```python
from build123d import *

# Parameters (mm, degrees)
SKETCH_1_W          = 62.2
SKETCH_1_H          = 78.2
SKETCH_1_W_2        = 59
SKETCH_1_H_2        = 75
EXTRUDE_1_DEPTH     = 30
SKETCH_2_W          = 62.2
SKETCH_2_H          = 78.2
EXTRUDE_1_2_DEPTH   = 1.6
SKETCH_3_W          = 5
SKETCH_3_H          = 5
EXTRUDE_2_DEPTH     = 3
SKETCH_4_W          = 1.5
SKETCH_4_H          = 5
EXTRUDE_3_DEPTH     = 1
SKETCH_5_W          = 1.5
SKETCH_5_H          = 5
SKETCH_5_H_2        = 4.722364884
EXTRUDE_4_DEPTH     = 1
FILLET_1_R          = 1
FILLET_2_R          = 1.8
SKETCH_6_R          = 2.2
CUT_EXTRUDE_1_DEPTH = 58.468078096
EXTRUDE_START       = 2
SKETCH_7_R          = 4
SKETCH_7_R_2        = 2.2
EXTRUDE_5_DEPTH     = 2
CHAMFER_1_SIZE      = 1.5
FILLET_3_R          = 1
CUT_EXTRUDE_2_REACH = 91.345


with BuildPart() as part:
    # Эскиз1 → Extrude 1 (new body)
    with BuildSketch(Plane.XY):
        Rectangle(SKETCH_1_W, SKETCH_1_H)
        Rectangle(SKETCH_1_W_2, SKETCH_1_H_2, mode=Mode.SUBTRACT)
    extrude(amount=EXTRUDE_1_DEPTH)

    # Эскиз2 → Extrude 1 2 (add)
    with BuildSketch(Plane.XY.offset(30)):
        Rectangle(SKETCH_2_W, SKETCH_2_H)
    extrude(amount=-EXTRUDE_1_2_DEPTH)

    # Эскиз3 → Бобышка-Вытянуть2 (add)
    with BuildSketch(Plane(origin=(0, 0, 28.4), x_dir=(-1, 0, 0), z_dir=(0, 0, -1))):
        with Locations((-27, 35)):
            Rectangle(SKETCH_3_W, SKETCH_3_H)
        with Locations((27, 35)):
            Rectangle(SKETCH_3_W, SKETCH_3_H)
        with Locations((-27, -35)):
            Rectangle(SKETCH_3_W, SKETCH_3_H)
        with Locations((27, -35)):
            Rectangle(SKETCH_3_W, SKETCH_3_H)
    extrude(amount=EXTRUDE_2_DEPTH)

    # Эскиз4 → Бобышка-Вытянуть3 (add)
    with BuildSketch(Plane.ZY.offset(-29.5)):
        with Locations((23.15, 35)):
            Rectangle(SKETCH_4_W, SKETCH_4_H)
        with Locations((23.15, -35)):
            Rectangle(SKETCH_4_W, SKETCH_4_H)
    extrude(amount=EXTRUDE_3_DEPTH)

    # Эскиз5 → Бобышка-Вытянуть4 (add)
    with BuildSketch(Plane(origin=(-29.5, 0, 0), x_dir=(0, 0, -1), z_dir=(1, 0, 0))):
        with Locations((-23.15, 35)):
            Rectangle(SKETCH_5_W, SKETCH_5_H)
        with Locations((-23.15, -35.138817558)):
            Rectangle(SKETCH_5_W, SKETCH_5_H_2)
    extrude(amount=EXTRUDE_4_DEPTH)

    # Скругление1
    fillet_1_edges = [part.edges().sort_by_distance(p)[0] for p in [
        (27, 32.5, 28.4),
        (24.5, 35, 28.4),
        (27, 32.5, 25.4),
        (24.5, 35, 25.4),
        (-24.5, 35, 28.4),
        (-27, 32.5, 28.4),
        (-24.5, 35, 25.4),
        (-27, 32.5, 25.4),
        (24.5, -35, 28.4),
        (27, -32.5, 28.4),
        (24.5, -35, 25.4),
        (27, -32.5, 25.4),
        (-27, -32.5, 28.4),
        (-24.5, -35, 28.4),
        (-27, -32.5, 25.4),
        (-24.5, -35, 25.4),
    ]]
    fillet(fillet_1_edges, radius=FILLET_1_R)

    # Скругление2
    # the kernel refuses this fillet: 1.8 mm, written as the material it adds along each edge
    with BuildSketch(Plane(origin=(29.5, -41.531128874, 23.9), x_dir=(0, 0, 1), z_dir=(0, 1, 0))) as fillet_2_piece_1_section:
        with BuildLine():
            CenterArc((1.61245155, -1.8), FILLET_2_R, 90, 63.612200039)
            Line((0, -1), (0, 0))
            Line((0, 0), (1.61245155, 0))
        make_face()
    fillet_2_piece_1 = extrude(amount=9.031128874, mode=Mode.PRIVATE)
    fillet_2_piece_1 = split(fillet_2_piece_1, bisect_by=Plane(origin=(29.5, -39.1, 23.9), z_dir=(0, 1, 0)), keep=Keep.TOP, mode=Mode.PRIVATE)
    add(fillet_2_piece_1)
    with BuildSketch(Plane(origin=(-29.5, -32.777635116, 23.9), x_dir=(0, 0, 1), z_dir=(0, -1, 0))) as fillet_2_piece_2_section:
        with BuildLine():
            CenterArc((1.61245155, -1.8), FILLET_2_R, 90, 63.612200039)
            Line((0, -1), (0, 0))
            Line((0, 0), (1.61245155, 0))
        make_face()
    fillet_2_piece_2 = extrude(amount=8.753493758, mode=Mode.PRIVATE)
    fillet_2_piece_2 = split(fillet_2_piece_2, bisect_by=Plane(origin=(-29.5, -39.1, 23.9), z_dir=(0, 1, 0)), keep=Keep.TOP, mode=Mode.PRIVATE)
    add(fillet_2_piece_2)
    with BuildSketch(Plane(origin=(-29.5, 41.531128874, 23.9), x_dir=(0, 0, 1), z_dir=(0, -1, 0))) as fillet_2_piece_3_section:
        with BuildLine():
            CenterArc((1.61245155, -1.8), FILLET_2_R, 90, 63.612200039)
            Line((0, -1), (0, 0))
            Line((0, 0), (1.61245155, 0))
        make_face()
    fillet_2_piece_3 = extrude(amount=9.031128874, mode=Mode.PRIVATE)
    fillet_2_piece_3 = split(fillet_2_piece_3, bisect_by=Plane(origin=(-29.5, 39.1, 23.9), z_dir=(0, -1, 0)), keep=Keep.TOP, mode=Mode.PRIVATE)
    add(fillet_2_piece_3)
    with BuildSketch(Plane(origin=(29.5, 41.531128874, 23.9), x_dir=(0, 0, 1), z_dir=(0, -1, 0))) as fillet_2_piece_4_section:
        with BuildLine():
            CenterArc((1.61245155, 1.8), FILLET_2_R, 206.387799961, 63.612200039)
            Line((0, 1), (0, 0))
            Line((0, 0), (1.61245155, 0))
        make_face()
    fillet_2_piece_4 = extrude(amount=9.031128874, mode=Mode.PRIVATE)
    fillet_2_piece_4 = split(fillet_2_piece_4, bisect_by=Plane(origin=(29.5, 39.1, 23.9), z_dir=(0, -1, 0)), keep=Keep.TOP, mode=Mode.PRIVATE)
    add(fillet_2_piece_4)

    # Эскиз6 → Вырез-Вытянуть1 (cut, through all)
    with BuildSketch(Plane(origin=(0, 0, 28.4), x_dir=(-1, 0, 0), z_dir=(0, 0, -1))):
        with Locations((-19.5, 25)):
            Circle(SKETCH_6_R)
        with Locations((0.5, 25)):
            Circle(SKETCH_6_R)
        with Locations((0.5, -25)):
            Circle(SKETCH_6_R)
        with Locations((-19.5, -25)):
            Circle(SKETCH_6_R)
    extrude(amount=-CUT_EXTRUDE_1_DEPTH, mode=Mode.SUBTRACT)

    # Эскиз7 → Бобышка-Вытянуть5 (add)
    # profile 1 of 4: a face of its own
    with BuildSketch(Plane(origin=(0, 0, 28.4), x_dir=(-1, 0, 0), z_dir=(0, 0, -1)).offset(EXTRUDE_START)):
        with Locations(Location((-19.5, 25, 0), (0, 0, 180))):
            Circle(SKETCH_7_R)
        with Locations((-19.5, 25)):
            Circle(SKETCH_7_R_2, mode=Mode.SUBTRACT)
    # profile 2 of 4: a face of its own
    with BuildSketch(Plane(origin=(0, 0, 28.4), x_dir=(-1, 0, 0), z_dir=(0, 0, -1)).offset(EXTRUDE_START)):
        with Locations(Location((0.5, 25, 0), (0, 0, 180))):
            Circle(SKETCH_7_R)
        with Locations((0.5, 25)):
            Circle(SKETCH_7_R_2, mode=Mode.SUBTRACT)
    # profile 3 of 4: a face of its own
    with BuildSketch(Plane(origin=(0, 0, 28.4), x_dir=(-1, 0, 0), z_dir=(0, 0, -1)).offset(EXTRUDE_START)):
        with Locations(Location((-19.5, -25, 0), (0, 0, 180))):
            Circle(SKETCH_7_R)
        with Locations((-19.5, -25)):
            Circle(SKETCH_7_R_2, mode=Mode.SUBTRACT)
    # profile 4 of 4: a face of its own
    with BuildSketch(Plane(origin=(0, 0, 28.4), x_dir=(-1, 0, 0), z_dir=(0, 0, -1)).offset(EXTRUDE_START)):
        with Locations(Location((0.5, -25, 0), (0, 0, 180))):
            Circle(SKETCH_7_R)
        with Locations((0.5, -25)):
            Circle(SKETCH_7_R_2, mode=Mode.SUBTRACT)
    extrude(amount=-EXTRUDE_5_DEPTH)

    # Фаска1
    chamfer_1_edges = [part.edges().sort_by_distance(p)[0] for p in [
        (21.7, 25, 26.4),
        (1.7, 25, 26.4),
        (21.7, -25, 26.4),
        (1.7, -25, 26.4),
    ]]
    chamfer(chamfer_1_edges, length=CHAMFER_1_SIZE)

    # Скругление3
    fillet_3_edges = [part.edges().sort_by_distance(p)[0] for p in [
        (31.1, -39.1, 15),
        (-31.1, -39.1, 15),
        (-31.1, 39.1, 15),
        (31.1, 39.1, 15),
    ]]
    fillet(fillet_3_edges, radius=FILLET_3_R)

    # Эскиз8 → Вырез-Вытянуть2 (cut, up to next)
    with BuildSketch(Plane(origin=(0, 39.1, 0), x_dir=(1, 0, 0), z_dir=(0, 1, 0)), mode=Mode.PRIVATE) as cut_extrude_2_sk1:
        with BuildLine():
            Line((18.995015929, -25.968474999), (14.239793371, -25.968474999))
            ThreePointArc((14.239793371, -25.968474999), (12.517359829, -24.246041457), (14.239793371, -22.523607914))
            Line((14.239793371, -22.523607914), (18.995015929, -22.523607914))
            ThreePointArc((18.995015929, -22.523607914), (20.717449472, -24.246041457), (18.995015929, -25.968474999))
        make_face()
    cut_extrude_2_tool1 = extrude(cut_extrude_2_sk1.sketch, amount=-CUT_EXTRUDE_2_REACH, mode=Mode.PRIVATE) & part.part
    add(cut_extrude_2_tool1.solids().sort_by_distance((16.617405, 39.1, 24.246041))[0], mode=Mode.SUBTRACT)


solid = part.part
```
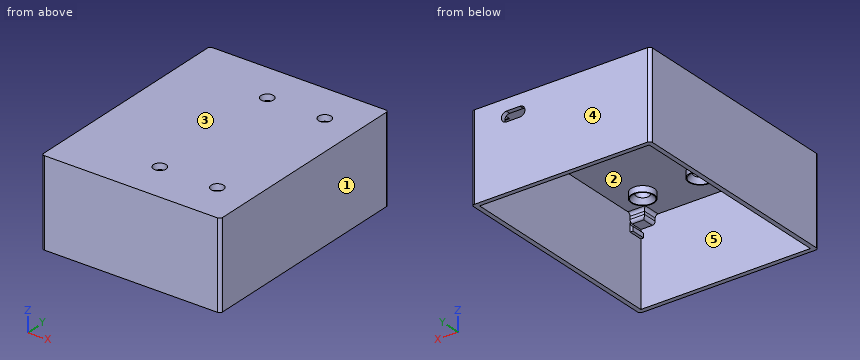
Verification items for the finished model (mm, model axes). Face numbers are marked on the shaded views. A direction names the side the tool comes from. Round coordinates to 2 decimals unless told otherwise and drop trailing zeros. Write each loop counter-clockwise with the first axis right and the second up, starting at its lowest first coordinate (ties: lowest second). Pieces come first, ordered by that corner, then holes.
1. Draft check along Y on the marked faces 3, 4 and 5. Enter one of: +Y half, -Y half, draft (parallel to the pull), parting line (faces both ways), or undercut.
2. Gauge pin test, flat ends, axial feed: P1, Ø2.5, axis at x = 19.5, y = -25, coming from the -Z side; P2, Ø0.5, axis at x = 29, y = 34, coming from the -Z side; P3, Ø4, axis at x = -0.5, y = -25.5, coming from the -Z side. Record the tip position at first contact, or that the pin passes through.
3. Section check B-B on x = -0.5. Enter the section's corners in (y, z), plus the area to 3 significant figures.
4. Scan lines: L1, parallel to Y at x = 19.5, z = 29.5; L2, parallel to X at y = -25.5, z = 12.25; L3, parallel to Y at x = -16, z = 10.25. Record each from-to range of solid material in increasing order.
5. Section check D-D on x = -13. Enter the section's corners in (y, z), plus the area to 3 significant figures.
6. Section check C-C on z = 20. Enter the section's corners in (x, y), plus the area to 3 significant figures.
7. Section check A-A on y = -25. Enter the section's corners in (x, z), plus the area to 3 significant figures.
8. Access from +Z, -Z, +X, -X, +Y, -Y to the whole of each face (thin tool, end or side, straight path). Record for the marked faces 1 and 2.
Answer:
1. face 3: draft
1. face 4: +Y half
1. face 5: undercut
2. P1: passes through
2. P2: stops at z = 22.4
2. P3: stops at z = 27.6
3. outline: (-39.1, 0) - (-37.5, 0) - (-37.5, 28.4) - (-29, 28.4) - (-29, 26.4) - (-28.7, 26.4) - (-27.2, 27.9) - (-27.2, 30) - (-39.1, 30) - close; (-22.8, 27.9) - (-21.3, 26.4) - (-21, 26.4) - (-21, 28.4) - (21, 28.4) - (21, 26.4) - (21.3, 26.4) - (22.8, 27.9) - (22.8, 30) - (-22.8, 30) - close; (27.2, 27.9) - (28.7, 26.4) - (29, 26.4) - (29, 28.4) - (37.5, 28.4) - (37.5, 0) - (39.1, 0) - (39.1, 30) - (27.2, 30) - close
3. area: 212 mm2
4. L1: y = -39.1 to -27.2, -22.8 to 22.8, 27.2 to 39.1
4. L2: x = -31.1 to -29.5, 29.5 to 31.1
4. L3: y = -39.1 to -37.5, 37.5 to 39.1
5. outline: (-39.1, 0) - (-37.5, 0) - (-37.5, 28.4) - (37.5, 28.4) - (37.5, 0) - (39.1, 0) - (39.1, 30) - (-39.1, 30) - close
5. area: 216 mm2
6. outline: (-31.1, -38.1) arc R1 ccw to (-30.1, -39.1) - (30.1, -39.1) arc R1 ccw to (31.1, -38.1) - (31.1, 38.1) arc R1 ccw to (30.1, 39.1) - (-30.1, 39.1) arc R1 ccw to (-31.1, 38.1) - close; hole (-29.5, -37.5) - (29.5, -37.5) - (29.5, 37.5) - (-29.5, 37.5) - close
6. area: 438 mm2
7. outline: (-31.1, 0) - (-29.5, 0) - (-29.5, 28.4) - (-4.5, 28.4) - (-4.5, 26.4) - (-4.2, 26.4) - (-2.7, 27.9) - (-2.7, 30) - (-31.1, 30) - close; (1.7, 27.9) - (3.2, 26.4) - (3.5, 26.4) - (3.5, 28.4) - (15.5, 28.4) - (15.5, 26.4) - (15.8, 26.4) - (17.3, 27.9) - (17.3, 30) - (1.7, 30) - close; (21.7, 27.9) - (23.2, 26.4) - (23.5, 26.4) - (23.5, 28.4) - (29.5, 28.4) - (29.5, 0) - (31.1, 0) - (31.1, 30) - (21.7, 30) - close
7. area: 186 mm2
8. face 1: +Z, -Z, +X, +Y, -Y
8. face 2: -Z
